```python
from build123d import *

# Parameters (mm, degrees)
SKETCH_1_W           = 10
SKETCH_1_H           = 8.5
EXTRUDE_1_DEPTH      = 10
CUT_EXTRUDE_1_DEPTH  = 8.5
EXTRUDE_2_DEPTH      = 4
EXTRUDE_2_DEPTH_BACK = 9
SKETCH_3_W           = 1
SKETCH_3_H           = 1


with BuildPart() as part:
    # 草图1 → 拉伸1 (new body)
    with BuildSketch(Plane(origin=(0, 0, 0), x_dir=(1, 0, 0), z_dir=(0, 1, 0))):
        Rectangle(SKETCH_1_W, SKETCH_1_H)
    extrude(amount=EXTRUDE_1_DEPTH)

    # 草图2 → 切除-拉伸1 (cut)
    with BuildSketch(Plane(origin=(0, 10, 0), x_dir=(-1, 0, 0), z_dir=(0, 1, 0))):
        Polygon((-5, 1.75), (-5, 4.25), (5, 4.25), (5, -4.25), (-5, -4.25), (-5, -1.75), (-2, -1.75), (-2, 1.75), align=None)
    extrude(amount=-CUT_EXTRUDE_1_DEPTH, mode=Mode.SUBTRACT)

    # 草图3 → 拉伸2 (add, two sides: drawn at the far end of the back side and taken through both)
    with BuildSketch(Plane.XZ.offset(-EXTRUDE_2_DEPTH_BACK)):
        with Locations((0, 1.905)):
            Rectangle(SKETCH_3_W, SKETCH_3_H)
        with Locations((0, -1.905)):
            Rectangle(SKETCH_3_W, SKETCH_3_H)
    extrude(amount=EXTRUDE_2_DEPTH + EXTRUDE_2_DEPTH_BACK)


solid = part.part
```
Here's how the part is built. I have some questions about the finished solid (model axes, mm). A direction names the side the tool comes from. Coordinates: 2 decimals unless noted, no trailing zeros. Order: outer loops, then holes, each group sorted by start corner. A loop starts at its lowest first (then second) coordinate and runs counter-clockwise, first axis right, second up. Notation, with made-up numbers: (73, 7.25) - (112, 7.25) arc R10 ccw to (112, 24.25) - close; hole circle Ø8 at (67.25, 8). An arc over 180 degrees is marked (long way). One line per question, with ' | ' between items. Start each with the question number.
1. If we section it at D-D (z = -1.25): Write out the boundary of the cut face in (x, y), and give its area (3 significant figures).
2. If we mould it in two halves opening along X, with no side actions, what happens to faces 4 (the flat face through (0.5, 5, -2)), 5 (the flat face through (-0.5, 5, 2)), 6 (the flat face through (0, -4, -2))? For each: released by +X, released by -X, zero draft, split by the parting line, or undercut.
3. If we section it at B-B (y = 7.5): Write out the boundary of the cut face in (x, z) (3 decimals), and give its area (3 significant figures).
4. If we section it at C-C (x = 3.25): Write out the boundary of the cut face in (y, z).
5. I'm going to push flat-ended pins straight in: pin 1 Ø0.8 at (y, z) = (-1, 2) entering from +X; pin 2 Ø1.5 at (x, y) = (-3, 8) entering from -Z; pin 3 Ø0.8 at (y, z) = (-2, 2) entering from -X; pin 4 Ø0.9 at (x, y) = (3.5, 5) entering from +Z. Where does each tip first touch, or does it pass through?
6. Which directions (+Z, -Z, +X, -X, +Y, -Y) give clear straight access to the entire face, cutting with the end or side of a thin tool? Please do faces 1 (the flat face through (0.5, -2, -2)), 2 (the flat face through (3, 6, 1.75)), 3 (the flat face through (0, 5, -2.405)).
7. If we section it at A-A (y = -1): Write out the boundary of the cut face in (x, z) (3 decimals), and give its area (3 significant figures).
8. Please list where these lines run through material, in increasing order: line 1 along X through (y, z) = (1.75, -1.5); line 2 along Z through (x, y) = (2.75, 7); line 3 along Y through (x, z) = (0.75, 2). Write a range as [from, to].
Model answer:
1) outline: (-5, 0) - (5, 0) - (5, 10) - (2, 10) - (2, 1.5) - (-5, 1.5) - close | area: 40.5 mm²
2) face 4: undercut | face 5: released by -X | face 6: zero draft
3) outline: (-0.5, -2.405) - (0.5, -2.405) - (0.5, -1.405) - (-0.5, -1.405) - close; (-0.5, 1.405) - (0.5, 1.405) - (0.5, 2.405) - (-0.5, 2.405) - close; (2, -1.75) - (5, -1.75) - (5, 1.75) - (2, 1.75) - close | area: 12.5 mm²
4) outline: (0, -4.25) - (1.5, -4.25) - (1.5, -1.75) - (10, -1.75) - (10, 1.75) - (1.5, 1.75) - (1.5, 4.25) - (0, 4.25) - close
5) pin 1: stops at x = 0.5 | pin 2: passes through | pin 3: stops at x = -0.5 | pin 4: stops at z = 1.75
6) face 1: +Z, -Z, +X, -Y | face 2: +Z, +X, +Y | face 3: -Z, +X, -X, +Y
7) outline: (-0.5, -2.405) - (0.5, -2.405) - (0.5, -1.405) - (-0.5, -1.405) - close; (-0.5, 1.405) - (0.5, 1.405) - (0.5, 2.405) - (-0.5, 2.405) - close | area: 2.00 mm²
8) line 1: x = [-0.5, 0.5], [2, 5] | line 2: z = [-1.75, 1.75] | line 3: y = [0, 1.5]
